Read the model definition and answer for the solid it produces. Units are mm, in the model's axes. A direction names the side the tool comes from. Round coordinates to 2 decimals unless told otherwise and drop trailing zeros. Loops run counter-clockwise (first coordinate to the right, second up) from the corner with the lowest first, then second, coordinate; pieces in that order, holes last. Notation, with made-up numbers: (-19.5, 33) -> (-3.5, 33) arc R21 ccw to (-3.5, 68) -> close; hole circle Ø5 at (77.25, 83). An arc over 180 degrees is marked (long way). Put each result on its own line as item: value.
from build123d import *

# Parameters (mm, degrees)
SKETCH1_R           = 6
BOSS_EXTRUDE1_DEPTH = 38
SKETCH2_R           = 4.5
BOSS_EXTRUDE2_DEPTH = 12
BOSS_EXTRUDE3_DEPTH = 8
SKETCH4_R           = 3
BOSS_EXTRUDE4_DEPTH = 8
SKETCH5_R           = 4.5
CUT_EXTRUDE1_DEPTH  = 27
CUT_EXTRUDE2_DEPTH  = 5
SKETCH7_R           = 2.5
BOSS_EXTRUDE5_DEPTH = 12
SKETCH9_W           = 12
SKETCH9_H           = 1
CUT_EXTRUDE3_DEPTH  = 3.5


with BuildPart() as part:
    # Sketch1 → Boss-Extrude1 (new body)
    with BuildSketch(Plane.XY):
        Circle(SKETCH1_R)
    extrude(amount=BOSS_EXTRUDE1_DEPTH)

    # Sketch2 → Boss-Extrude2 (add)
    with BuildSketch(Plane(origin=(0, 0, 0), x_dir=(-1, 0, 0), z_dir=(0, 0, -1))):
        with Locations(Location((0, 0, 0), (0, 0, 180))):
            Circle(SKETCH2_R)
    extrude(amount=BOSS_EXTRUDE2_DEPTH)

    # Sketch3 → Boss-Extrude3 (add)
    with BuildSketch(Plane.XY.offset(38)):
        with BuildLine():
            ThreePointArc((-12.649110641, -3), (0, -13), (12.649110641, -3))
            ThreePointArc((12.649110641, -3), (6.302186147, 4.007182978), (2.649110641, 12.727223295))
            ThreePointArc((2.649110641, 12.727223295), (0, 13), (-2.649110641, 12.727223295))
            ThreePointArc((-2.649110641, 12.727223295), (-6.302186147, 4.007182978), (-12.649110641, -3))
        make_face()
    extrude(amount=-BOSS_EXTRUDE3_DEPTH)

    # Sketch4 → Boss-Extrude4 (add)
    with BuildSketch(Plane.XY.offset(38)):
        with Locations((0, 9)):
            Circle(SKETCH4_R)
    extrude(amount=BOSS_EXTRUDE4_DEPTH)

    # Sketch5 → Cut-Extrude1 (cut)
    with BuildSketch(Plane.XY.offset(38)):
        Circle(SKETCH5_R)
    extrude(amount=-CUT_EXTRUDE1_DEPTH, mode=Mode.SUBTRACT)

    # Sketch6 → Cut-Extrude2 (cut)
    with BuildSketch(Plane(origin=(-4.242640687, 4.242640687, 0), x_dir=(0, 0, -1), z_dir=(-0.7071067811865438, 0.7071067811865512, 0))):
        with BuildLine():
            Line((-19, 4), (-15, 4))
            ThreePointArc((-15, 4), (-11, 0), (-15, -4))
            Line((-15, -4), (-19, -4))
            ThreePointArc((-19, -4), (-23, 0), (-19, 4))
        make_face()
    extrude(amount=-CUT_EXTRUDE2_DEPTH, mode=Mode.SUBTRACT)

    # Sketch7 → Boss-Extrude5 (add)
    with BuildSketch(Plane(origin=(0, 0, -12), x_dir=(-1, 0, 0), z_dir=(0, 0, -1))):
        Circle(SKETCH7_R)
    extrude(amount=BOSS_EXTRUDE5_DEPTH)

    # Sketch9 → Cut-Extrude3 (cut, symmetric)
    with BuildSketch(Plane(origin=(0, 0, 0), x_dir=(0, 0, -1), z_dir=(1, 0, 0))):
        with Locations((6, 4)):
            Rectangle(SKETCH9_W, SKETCH9_H)
    extrude(amount=CUT_EXTRUDE3_DEPTH, both=True, mode=Mode.SUBTRACT)


solid = part.part
Item 1: The part is cut by section B-B (z = -9.5). Determine the outline of the cut face in (x, y).
Derived:
outline: (-2.83, 3.5) arc R4.5 ccw (long way) to (2.83, 3.5) -> close
Item 2: The part is cut by section D-D (z = 4). Determine the outline of the cut face in (x, y), then the cut area to 3 significant figures.
Derived:
outline: circle Ø12 at (0, 0)
area: 113 mm^2
Item 3: The part is cut by section C-C (z = 26). Determine the outline of the cut face in (x, y).
Derived:
outline: circle Ø12 at (0, 0); hole circle Ø9 at (0, 0)
Item 4: Which of the six approach directions +Z, -Z, +X, -X, +Y, -Y give full straight-line access (tool end or side, diameter ignored) to faces 4 (the cylindrical face through (2.769, -5.323, 14.79)), 5 (the cylindrical face through (-3.55, 3.43, 11)), 6 (the cylindrical face through (-3, 9, 42))?
Derived:
face 4: -Z
face 5: none
face 6: +Z
Item 5: The part is cut by section A-A (y = 7.25). Determine the outline of the cut face in (x, z).
Derived:
outline: (-4.53, 30) -> (4.53, 30) -> (4.53, 38) -> (2.44, 38) -> (2.44, 46) -> (-2.44, 46) -> (-2.44, 38) -> (-4.53, 38) -> close
Item 6: Find the intervals of material crossed by line 1 along Z through (x, y) = (3.25, 1); line 2 along Y through (x, z) = (0, 25.5); line 3 along Z through (x, y) = (-5.75, 2.75), in increasing order.
Derived:
line 1: z = -12 to 11
line 2: y = -6 to -4.5, 4.5 to 6
line 3: z = 30 to 38
Item 7: Flat-ended cylindrical pins translate along their axes: pin 1 Ø3 at (y, z) = (-2.5, 13.5) entering from -X; pin 2 Ø6 at (y, z) = (4, 26) entering from +X; pin 3 Ø2 at (x, y) = (-8, -3.5) entering from -Z; pin 4 Ø13 at (x, y) = (-1.5, -2.5) entering from -Z. Find the tip coordinate at first contact, or state that the pin passes through.
Derived:
pin 1: stops at x = -5.92
pin 2: stops at x = 5.92
pin 3: stops at z = 30
pin 4: stops at z = -24
Item 8: For a pull along Z with two mould halves and no side action, classify faces 1 (the flat face through (0.506, 5.15, 16.972)), 2 (the flat face through (0, 3.5, -6)), 3 (the flat face through (0, 4, 0)) as pulls with the +Z half, pulls with the -Z half, needs draft (parallel to the pull), parting line crosses it, or undercut.
Derived:
face 1: undercut
face 2: needs draft
face 3: pulls with the -Z half
